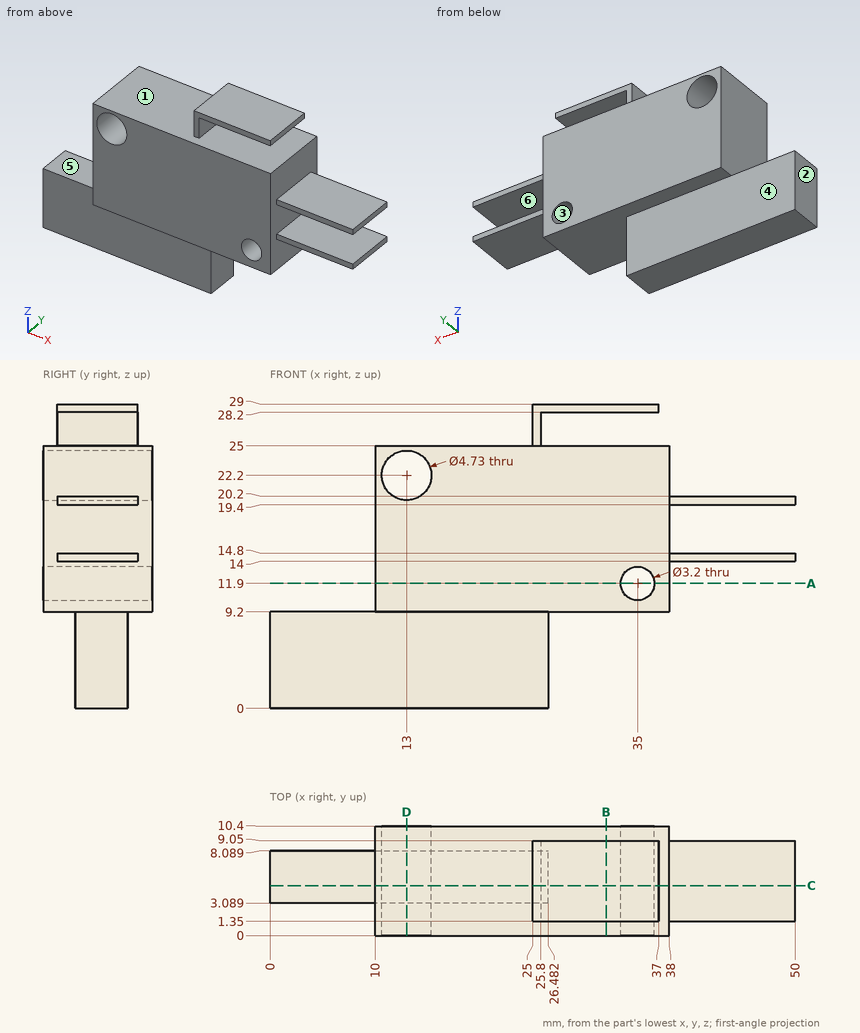
Print and shaded views of the part. All mm, measured from the part's lowest x, y and z. A direction names the side the tool comes from. Give positions to 0.01 mm unless a question says otherwise; leave off trailing zeros. Write each loop counter-clockwise with the first axis right and the second up, starting at its lowest first coordinate (ties: lowest second). Pieces come first, ordered by that corner, then holes. Notation, with made-up numbers: (-1, 12.5) - (50, 12.5) arc R23 ccw to (50, 25.5) - close; hole circle Ø1 at (2, 75). An arc over 180 degrees is marked (long way). Put each result on its own line as item: value.
(1) Wall check: L1, parallel to X at y = 5.75, z = 11.9; L2, parallel to X at y = 7.25, z = 22.2 (3 decimals); L3, parallel to Z at x = 48.5, y = 5.5. Give the ranges that are in metal, low to high.
Working result:
L1: 10 to 33.4, 36.6 to 38
L2: 10 to 10.635, 15.365 to 38
L3: 14 to 14.8, 19.4 to 20.2
(2) Drop flat-ended pins along their axis: pin 1 Ø2.5 at (x, y) = (45.5, 4) entering from -Z; pin 2 Ø0.9 at (x, z) = (46, 14.5) entering from -Y; pin 3 Ø0.9 at (x, z) = (46, 14.5) entering from +Y. Give the stop position or say it passes through.
Working result:
pin 1: z = 14
pin 2: y = 1.35
pin 3: y = 9.05
(3) Tool access for the marked faces 4, 5 and 6: list every direction of +Z, -Z, +X, -X, +Y, -Y with a clear straight run to the whole face (end or side of a thin tool).
Working result:
face 4: -Z, +X, -X, +Y
face 5: +Z, -X, +Y, -Y
face 6: +X, +Y, -Y
(4) Pull direction X, two halves, no side cores. Call the marked faces 1, 2 and 3: released by +X, released by -X, zero draft, split by the parting line, or undercut.
Working result:
face 1: zero draft
face 2: released by -X
face 3: undercut
(5) Saw through at A-A (z = 11.9). List the corners of the cut face in (x, y).
Working result:
outline: (10, 0) - (33.4, 0) - (33.4, 10.4) - (10, 10.4) - close; (36.6, 0) - (38, 0) - (38, 10.4) - (36.6, 10.4) - close
(6) Saw through at B-B (x = 32). List the corners of the cut face in (y, z).
Working result:
outline: (0, 9.2) - (10.4, 9.2) - (10.4, 25) - (0, 25) - close; (1.35, 28.2) - (9.05, 28.2) - (9.05, 29) - (1.35, 29) - close
(7) Saw through at C-C (y = 4.75). List the corners of the cut face in (x, z) (3 decimals), then the cut area to 3 significant figures.
Working result:
outline: (0, 0) - (26.482, 0) - (26.482, 9.2) - (38, 9.2) - (38, 14) - (50, 14) - (50, 14.8) - (38, 14.8) - (38, 19.4) - (50, 19.4) - (50, 20.2) - (38, 20.2) - (38, 25) - (25.8, 25) - (25.8, 28.2) - (37, 28.2) - (37, 29) - (25, 29) - (25, 25) - (10, 25) - (10, 9.2) - (0, 9.2) - close; hole circle Ø4.73 at (13, 22.2); hole circle Ø3.2 at (35, 11.9)
area: 692 mm^2
(8) Saw through at D-D (x = 13). List the corners of the cut face in (y, z) (3 decimals), then the cut area to 3 significant figures.
Working result:
outline: (0, 9.2) - (3.089, 9.2) - (3.089, 0) - (8.089, 0) - (8.089, 9.2) - (10.4, 9.2) - (10.4, 19.835) - (0, 19.835) - close; (0, 24.565) - (10.4, 24.565) - (10.4, 25) - (0, 25) - close
area: 161 mm^2
